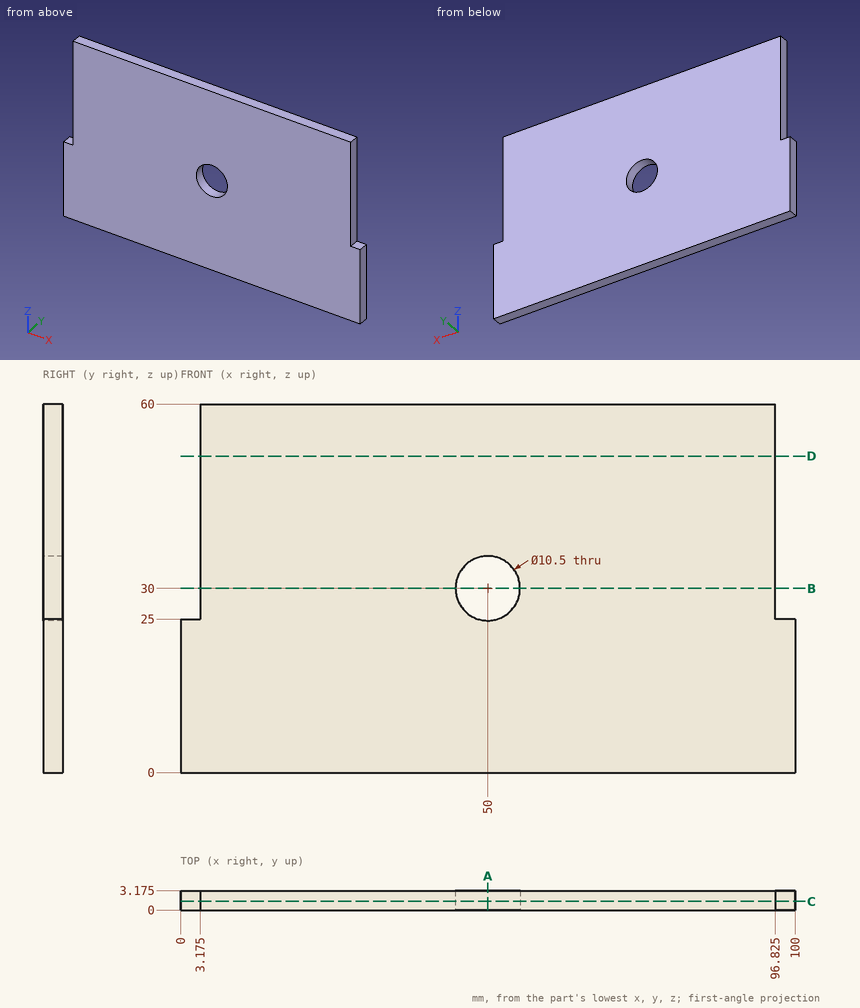
Source: three-view drawing plus pictorial views. Frame: mm from the lowest corner of the part. Give positions to 0.01 mm unless a question says otherwise; leave off trailing zeros. Write each loop counter-clockwise with the first axis right and the second up, starting at its lowest first coordinate (ties: lowest second). Pieces come first, ordered by that corner, then holes. Notation, with made-up numbers: (-15.75, 68.5) -> (34.25, 68.5) arc R18 ccw to (34.25, 72.5) -> close; hole circle Ø7 at (-32.75, 0.5). An arc over 180 degrees is marked (long way). Write item = value, one per line.
Q1. Cut plane D-D on z = 51.5. Return loops of the section in (x, y) (3 decimals), then the cut area to 3 significant figures.
Here are the results:
outline = (3.175, 0) -> (96.825, 0) -> (96.825, 3.175) -> (3.175, 3.175) -> close
area = 297 mm²
Q2. Cut plane A-A on x = 50. Return loops of the section in (y, z) (3 decimals).
Here are the results:
outline = (0, 0) -> (3.175, 0) -> (3.175, 24.75) -> (0, 24.75) -> close; (0, 35.25) -> (3.175, 35.25) -> (3.175, 60) -> (0, 60) -> close
Q3. Cut plane B-B on z = 30. Return loops of the section in (x, y) (3 decimals), then the cut area to 3 significant figures.
Here are the results:
outline = (3.175, 0) -> (44.75, 0) -> (44.75, 3.175) -> (3.175, 3.175) -> close; (55.25, 0) -> (96.825, 0) -> (96.825, 3.175) -> (55.25, 3.175) -> close
area = 264 mm²
Q4. Line query: line 1 (X direction, y = 0.6, z = 30) (3 decimals); line 2 (X direction, y = 0.2, z = 45) (3 decimals). Output: solid intervals per line, ascending. Write a range as from..to.
Here are the results:
line_1 = 3.175..44.75, 55.25..96.825
line_2 = 3.175..96.825
Q5. Cut plane C-C on y = 1.45. Return loops of the section in (x, z) (3 decimals).
Here are the results:
outline = (0, 0) -> (100, 0) -> (100, 25) -> (96.825, 25) -> (96.825, 60) -> (3.175, 60) -> (3.175, 25) -> (0, 25) -> close; hole circle Ø10.5 at (50, 30)
Q6. First-contact query: pin 1 (1 mm diameter, centred on y = 1, z = 34, fed in from -X) (3 decimals); pin 2 (1 mm diameter, centred on x = 2, y = 2.5, fed in from +Z); pin 3 (1 mm diameter, centred on y = 1.5, z = 36.5, fed in from +X) (3 decimals). Flat tips, straight axial feed; report the tip coordinate or a pass-through.
Here are the results:
pin_1 = 3.175
pin_2 = 25
pin_3 = 96.825
